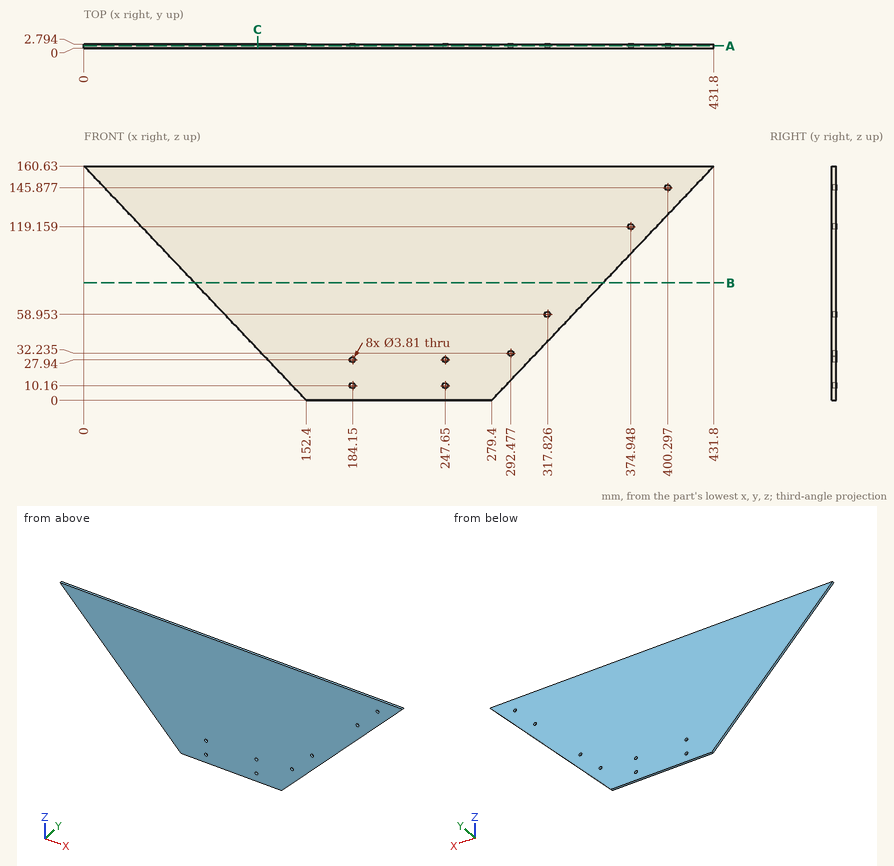
Check sheet for the drawn part. Datum: minimum x, y, z corner. Units: mm. Round coordinates to 2 decimals unless told otherwise and drop trailing zeros. Order: outer loops, then holes, each group sorted by start corner. A loop starts at its lowest first (then second) coordinate and runs counter-clockwise, first axis right, second up.
(1) Cross-section at B-B, the plane z = 80.5. Enter the section's corners in (x, y) (1 decimal).
(2) Cross-section at A-A, the plane y = 1.55. State how many separate pieces and enclosed holes the cut face has, and give its area (3 significant figures).
(3) Cross-section at C-C, the plane x = 119. Enter the section's corners in (y, z).
(4) Scan lines: probe 1 along Z at (x, y) = (184.15, 1.75) (1 decimal); probe 2 along X at (y, z) = (1.6, 10.16) (1 decimal); probe 3 along Z at (x, y) = (319, 2.75) (1 decimal). Record each from-to range of solid material in increasing order.
(5) Go/stop test with flat-tipped pins: P1, Ø3.5, axis at x = 247.65, z = 27.94, coming from the -Y side; P2, Ø6, axis at x = 184.15, z = 27.94, coming from the -Y side. Record where each tip stops, or that it passes through.
Check sheet entries:
1. outline: (76, 0) - (355.8, 0) - (355.8, 2.8) - (76, 2.8) - close
2. separate pieces: 1
2. enclosed holes: 8
2. area: 44,800 mm2
3. outline: (0, 35.2) - (2.79, 35.2) - (2.79, 160.63) - (0, 160.63) - close
4. probe 1: z = 0 to 8.3, 12.1 to 26, 29.8 to 160.6
4. probe 2: x = 142.8 to 182.2, 186.1 to 245.7, 249.6 to 289
4. probe 3: z = 41.7 to 57.5, 60.5 to 160.6
5. P1: passes through
5. P2: stops at y = 0
